Autodesk Inventor part; units mm, degrees
ref_plane "Plano de trabajo1" through (0, 33, 0) normal (0, 1, 0) x (-1, 0, 0)
ref_plane "YZ Plane" through (0, 0, 0) normal (1, 0, 0) x (0, 1, 0)
ref_plane "XY Plane" through (0, 0, 0) normal (0, 0, 1) x (1, 0, 0)
sketch "Boceto1" plane through (0, 0, 0) normal (0, 0, 1) x (1, 0, 0)
  line L0 (0, 100) -> (0, -100) construction
  line L1 (-100, 0) -> (100, 0) construction
  line L2 (-21, -50) -> (-21, 0)
  line L3 (21, -50) -> (21, 0)
  arc A0 (21, 0) -> (-21, 0) centre (0, 0) ccw
  arc A1 (33, 0) -> (-33, 0) centre (0, 0) ccw
  line L4 (-33, 0) -> (-33, -50)
  line L5 (33, 0) -> (33, -50)
  line L6 (-21, -50) -> (-33, -50)
  line L7 (21, -50) -> (33, -50)
  circle A2 centre (0, 48) radius 7.5
  arc A3 (13.9054, 53.625) -> (-13.9054, 53.625) centre (0, 48) ccw
  line L8 (-13.9054, 53.625) -> (-30.5918, 12.375)
  line L9 (13.9054, 53.625) -> (30.5918, 12.375)
  line L10 (-33, 0) -> (-57, 0)
  line L11 (-57, 0) -> (-57, 8)
  line L12 (-57, 8) -> (-32.0156, 8)
  line L13 (100, 0) -> (-100, 0) construction
  line L14 (33, 0) -> (57, 0)
  line L15 (57, 0) -> (57, 8)
  line L16 (57, 8) -> (32.0156, 8)
  point P0 (0, 33)
  dimension "d0" = 200
  dimension "d1" = 200
  dimension "d2" = 50
  dimension "d3" = 50
  dimension "d4" = 42
  dimension "d5" = 33
  dimension "d6" = 15
  dimension "d7" = 48
  dimension "d8" = 15
  dimension "d9" = 24
  dimension "d10" = 8
  dimension "d26" = 33
extrude "Extrusión1" add sketch "Boceto1" along normal blind 60 contours L6 L4 A1 L5 L7 L3 A0 L2
extrude "Extrusión2" add sketch "Boceto1" along normal blind 12 contours L8 A3 L9 A1
extrude "Extrusión3" add sketch "Boceto1" along normal blind 48 contours L10 L11 L12 A1 | A1 L16 L15 L14
fillet "Empalme1" radius 12 4 edges at (57, 4, 48) (-57, 4, 48) (57, 4, 0) (-57, 4, 0)
sketch "Boceto2" plane through (32.0156, 8, 48) normal (0, 1, 0) x (1, 0, 0)
  line L0 (12.9844, 0) -> (0, 0)
  line L1 (12.9844, 48) -> (0, 48)
  line L2 (0, 0) -> (0, 48)
  circle A0 centre (12, 36) radius 6
  circle A1 centre (12, 12) radius 6
  line L3 (-32.0156, 86.4506) -> (-32.0156, -39.8075) construction
  circle A2 centre (-76.0312, 36) radius 6
  circle A3 centre (-76.0312, 12) radius 6
  point P0 (-32.0156, 48)
  dimension "d18" = 12
  dimension "d19" = 12
  dimension "d20" = 12
  dimension "d21" = 12
  dimension "d22" = 12
  dimension "d23" = 12
extrude "Extrusión4" cut sketch "Boceto2" against normal blind 48
ref_plane "Plano de trabajo1" through (0, 33, 0) normal (0, 1, 0) x (-1, 0, 0)
sketch "Boceto3" plane through (0, 33, 0) normal (0, 1, 0) x (-1, 0, 0)
  line L0 (-17.465, 45) -> (17.465, 45)
  line L1 (17.465, 45) -> (17.465, 20)
  line L2 (17.465, 20) -> (-17.465, 20)
  line L3 (-17.465, 20) -> (-17.465, 45)
  line L4 (-17.465, 45) -> (17.465, 20) construction
  line L5 (17.465, 45) -> (-17.465, 20) construction
  line L6 (13.9054, 12) -> (-13.9054, 12)
  line L7 (0, -11.8316) -> (0, 73.0134) construction
  circle A0 centre (0, 32.5) radius 6
  point P0 (0, 0)
  dimension "d28" = 8
  dimension "d29" = 25
  dimension "d30" = 34.93
  dimension "d31" = 12
extrude "Extrusión5" cut sketch "Boceto3" against normal blind 5
extrude "Extrusión6" cut sketch "Boceto3" against normal blind 20 contours A0
properties material "Acero inoxidable"
The listing builds one solid part. Answer for the finished solid, in the listing's coordinates (mm). A direction names the side the tool comes from. Round coordinates to 2 decimals unless told otherwise and drop trailing zeros. Loops run counter-clockwise (first coordinate to the right, second up) from the corner with the lowest first, then second, coordinate; pieces in that order, holes last. Notation, with made-up numbers: (4.5, -37.5) - (61.5, -37.5) arc R23 ccw to (61.5, -14.5) - close; hole circle Ø4 at (75.5, 43). An arc over 180 degrees is marked (long way). Return JSON: item names as keys, results as strings. Group by question number.
1. Which of the six approach directions +Z, -Z, +X, -X, +Y, -Y give full straight-line access (tool end or side, diameter ignored) to faces 4 (the flat face through (45, 0, 24)), 5 (the flat face through (-33, -25, 30)), 6 (the flat face through (45, 8, 24)), 7 (the flat face through (-4, 28, 27)), 8 (the cylindrical face through (-0.73, 32.99, 49.58))?
2. The part is cut by section A-A on y = -13. Determine the outline of the cut face in (x, z).
3. Consider probe 1 along X at (y, z) = (-15, 47); probe 2 along Z at (x, y) = (44.5, 1); probe 3 along X at (y, z) = (3, 36). Determine where each line is inside the solid, lowest interval first.
4. The part is cut by section C-C on z = 32.5. Determine the outline of the cut face in (x, y), then the cut area to 3 significant figures.
5. The part is cut by section D-D on z = 40.5. Determine the outline of the cut face in (x, y), then the cut area to 3 significant figures.
6. Each of these flat-tipped pins is pushed along its axis until it touches: P1, Ø6, axis at y = -7, z = 34, coming from the +X side; P2, Ø3, axis at x = -37, y = 0.5, coming from the +Z side; P3, Ø15.5, axis at x = 44.02, z = 36, coming from the +Y side; P4, Ø6, axis at x = -30, y = -7.5, coming from the -Z side. Where does it stop, or does it pass through?
7. The part is cut by section B-B on x = 0. Determine the outline of the cut face in (y, z), then the cut area to 3 significant figures.
8. The mould has two halves that part along Z. Classify faces 1 (the cylindrical face through (-53.58, 4.06, 44.39)), 2 (the flat face through (-45, 0, 24)), 3 (the cylindrical face through (-38.473, 4.056, 38.298)): pulls with the +Z half, pulls with the -Z half, needs draft (parallel to the pull), parting line crosses it, or undercut.
Resolved:
{
 "1": {"face 4": "+Z, -Z, +X, -Y", "face 5": "+Z, -Z, -X, -Y", "face 6": "+Z, -Z, +X, +Y", "face 7": "+X, -X, +Y", "face 8": "+Z, +Y"},
 "2": {"outline": "(-33, 0) - (-21, 0) - (-21, 60) - (-33, 60) - close; (21, 0) - (33, 0) - (33, 60) - (21, 60) - close"},
 "3": {"probe 1": "x = -33 to -21, 21 to 33", "probe 2": "z = 0 to 6.02, 17.98 to 30.02, 41.98 to 48", "probe 3": "x = -57 to -50.02, -38.02 to -20.78, 20.78 to 38.02, 50.02 to 57"},
 "4": {"outline": "(-57, 0) - (-48.89, 0) - (-48.89, 8) - (-57, 8) - close; (-39.14, 0) - (-33, 0) - (-33, -50) - (-21, -50) - (-21, 0) arc R21 cw to (-6, 20.12) - (-6, 28) - (-17.46, 28) arc R33 ccw to (-32.02, 8) - (-39.14, 8) - close; (6, 20.12) arc R21 cw to (21, 0) - (21, -50) - (33, -50) - (33, 0) - (39.14, 0) - (39.14, 8) - (32.02, 8) arc R33 ccw to (17.46, 28) - (6, 28) - close; (48.89, 0) - (57, 0) - (57, 8) - (48.89, 8) - close", "area": "2,250 mm²"},
 "5": {"outline": "(-56.12, 0) - (-47.98, 0) - (-47.98, 8) - (-56.12, 8) - close; (-40.05, 0) - (-33, 0) - (-33, -50) - (-21, -50) - (-21, 0) arc R21 cw to (21, 0) - (21, -50) - (33, -50) - (33, 0) - (40.05, 0) - (40.05, 8) - (32.02, 8) arc R33 ccw to (17.46, 28) - (-17.46, 28) arc R33 ccw to (-32.02, 8) - (-40.05, 8) - close; (47.98, 0) - (56.12, 0) - (56.12, 8) - (47.98, 8) - close", "area": "2,350 mm²"},
 "6": {"P1": "stops at x = 33", "P2": "stops at z = 48", "P3": "stops at y = 8", "P4": "stops at z = 0"},
 "7": {"outline": "(21, 0) - (40.5, 0) - (40.5, 12) - (33, 12) - (33, 20) - (28, 20) - (28, 26.5) - (21, 26.5) - close; (21, 38.5) - (28, 38.5) - (28, 45) - (33, 45) - (33, 60) - (21, 60) - close; (55.5, 0) - (63, 0) - (63, 12) - (55.5, 12) - close", "area": "691 mm²"},
 "8": {"face 1": "pulls with the +Z half", "face 2": "needs draft", "face 3": "undercut"}
}
